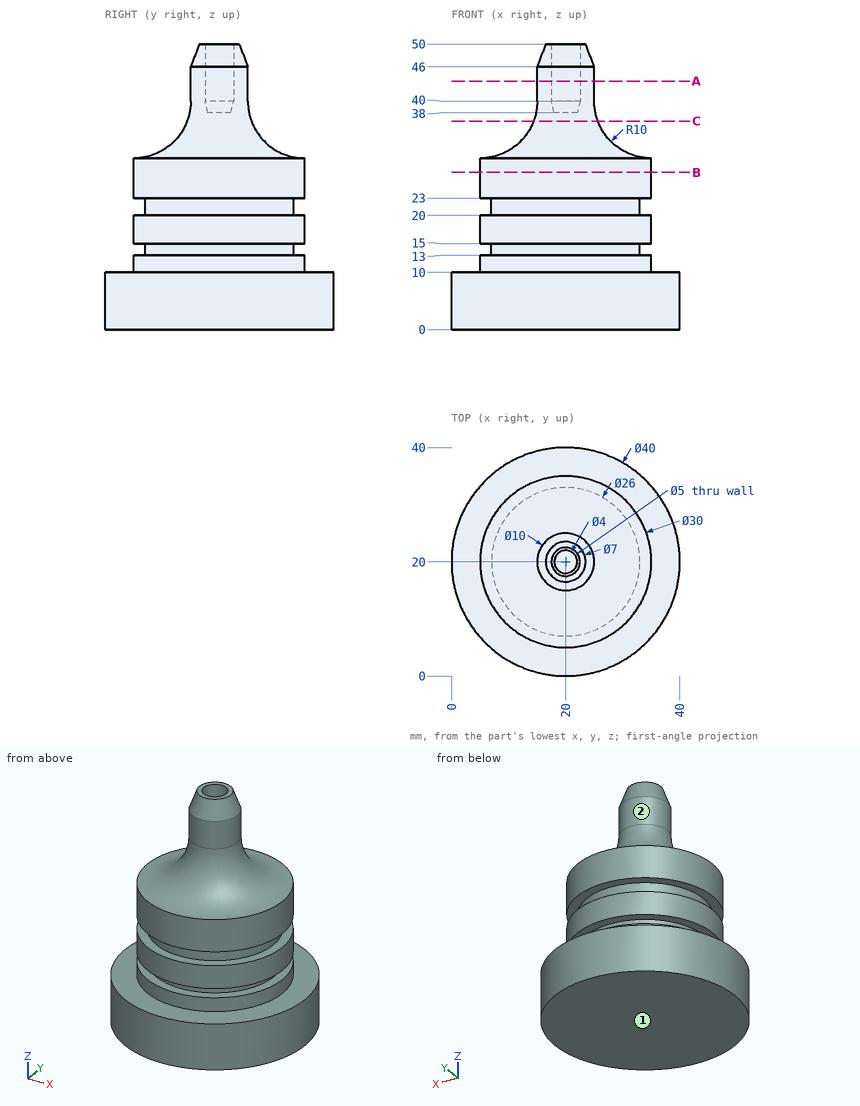
Geometry check sheet. Reference: drawing and pictorial views, mm from the part's lowest x, y, z. A direction names the side the tool comes from. Round coordinates to 2 decimals unless told otherwise and drop trailing zeros. Loops run counter-clockwise (first coordinate to the right, second up) from the corner with the lowest first, then second, coordinate; pieces in that order, holes last. Notation, with made-up numbers: M 64.25,62.5 L 91.25,62.5 A17 cw 91.25,79.5 Z; hole C -14,-32.5 d4. An arc over 180 degrees is marked long. One line per item, written item: value.
(1) Thickness scan on line 1 (Y direction, x = 20, z = 44); line 2 (Z direction, x = 26, y = 35); line 3 (X direction, y = 20.5, z = 44.5). Record the ranges inside material, lowest first.
Computed values:
line 1: y = 15 to 17.5, 22.5 to 25
line 2: z = 0 to 10
line 3: x = 15.03 to 17.55, 22.45 to 24.97
(2) Access from +Z, -Z, +X, -X, +Y, -Y to the whole of each face (thin tool, end or side, straight path). Record for the marked faces 1 and 2.
Computed values:
face 1: -Z, +X, -X, +Y, -Y
face 2: +Z
(3) Sectioned sample at B-B, the plane z = 27.5. Record the cut outline in (x, y), then the cut area to 3 significant figures.
Computed values:
outline: C 20,20 d30
area: 707 mm^2
(4) Depth check by flat-ended pin: pin 1 Ø1.5 at (x, y) = (29, 24.5) entering from +Z (3 decimals); pin 2 Ø24 at (x, y) = (23, 13) entering from -Z; pin 3 Ø1.5 at (x, z) = (25, 33.5) entering from +Y; pin 4 Ø8 at (x, z) = (18.5, 7.5) entering from +Y. Enter the tip coordinate at first touch or a pass-through.
Computed values:
pin 1: stops at z = 31.775
pin 2: stops at z = 0
pin 3: stops at y = 26.54
pin 4: stops at y = 40
(5) Sectioned sample at A-A, the plane z = 43.5. Record the cut outline in (x, y).
Computed values:
outline: C 20,20 d10; hole C 20,20 d5
(6) Sectioned sample at C-C, the plane z = 36.5. Record the cut outline in (x, y) (1 decimal).
Computed values:
outline: C 20,20 d11.3
